```python
from build123d import *

# Parameters (mm, degrees)
SKETCH_3_W          = 4.4
SKETCH_3_H          = 18.2
EXTRUDE_1_DEPTH     = 1
SKETCH_4_R          = 0.95
CUT_EXTRUDE_1_DEPTH = 0.5
SKETCH_5_W          = 1
SKETCH_5_H          = 18.2
EXTRUDE_2_DEPTH     = 7
SKETCH_6_W          = 8.5
SKETCH_6_H          = 18.2
SKETCH_6_R          = 2
EXTRUDE_3_DEPTH     = 1
SKETCH_8_W          = 8.5
SKETCH_8_H          = 0.3
CUT_EXTRUDE_3_DEPTH = 0.2
SKETCH_9_R          = 0.6
CUT_EXTRUDE_4_DEPTH = 24.107989665
SKETCH_10_W         = 1
SKETCH_10_H         = 5.3
CUT_EXTRUDE_5_DEPTH = 2
FILLET_1_R          = 0.5


with BuildPart() as part:
    # 草圖3 → 填料-伸長1 (new body)
    with BuildSketch(Plane.XY):
        with Locations((3.460771452, 7.885973071)):
            Rectangle(SKETCH_3_W, SKETCH_3_H)
    extrude(amount=EXTRUDE_1_DEPTH)

    # 草圖4 → 除料-伸長1 (cut)
    with BuildSketch(Plane.XY.offset(1)):
        with Locations((3.460771452, 15.485973071)):
            Circle(SKETCH_4_R)
        with Locations((3.460771452, 0.285973071)):
            Circle(SKETCH_4_R)
        with Locations((3.460771452, 12.985973071)):
            Circle(SKETCH_4_R)
        with Locations((3.460771452, 2.785973071)):
            Circle(SKETCH_4_R)
    extrude(amount=-CUT_EXTRUDE_1_DEPTH, mode=Mode.SUBTRACT)

    # 草圖5 → 填料-伸長2 (add)
    with BuildSketch(Plane.XY.offset(1)):
        with Locations((5.160771452, 7.885973071)):
            Rectangle(SKETCH_5_W, SKETCH_5_H)
    extrude(amount=EXTRUDE_2_DEPTH)

    # 草圖6 → 填料-伸長3 (add)
    with BuildSketch(Plane.XY.offset(8)):
        with Locations((8.910771452, 7.885973071)):
            Rectangle(SKETCH_6_W, SKETCH_6_H)
        with Locations((9.254845598, 7.885973071)):
            Circle(SKETCH_6_R, mode=Mode.SUBTRACT)
    extrude(amount=EXTRUDE_3_DEPTH)

    # 草圖8 → 除料-伸長3 (cut)
    with BuildSketch(Plane.XY.offset(9)):
        with Locations((8.910771452, 7.885973071)):
            Rectangle(SKETCH_8_W, SKETCH_8_H)
    extrude(amount=-CUT_EXTRUDE_3_DEPTH, mode=Mode.SUBTRACT)

    # 草圖9 → 除料-伸長4 (cut, through all)
    with BuildSketch(Plane.XY.offset(0.5)):
        with Locations((3.460771452, 15.485973071)):
            Circle(SKETCH_9_R)
        with Locations((3.460771452, 12.985973071)):
            Circle(SKETCH_9_R)
        with Locations((3.460771452, 2.785973071)):
            Circle(SKETCH_9_R)
        with Locations((3.460771452, 0.285973071)):
            Circle(SKETCH_9_R)
    extrude(amount=-CUT_EXTRUDE_4_DEPTH, mode=Mode.SUBTRACT)

    # 草圖10 → 除料-伸長5 (cut)
    with BuildSketch(Plane.ZY.offset(-1.260771452)):
        with Locations((0.5, 7.885973071)):
            Rectangle(SKETCH_10_W, SKETCH_10_H)
    extrude(amount=-CUT_EXTRUDE_5_DEPTH, mode=Mode.SUBTRACT)

    # 圓角1
    fillet_1_edges = [part.edges().sort_by_distance(p)[0] for p in [
        (3.260771452, 5.235973071, 0.5),
        (3.260771452, 10.535973071, 0.5),
    ]]
    fillet(fillet_1_edges, radius=FILLET_1_R)


solid = part.part
```
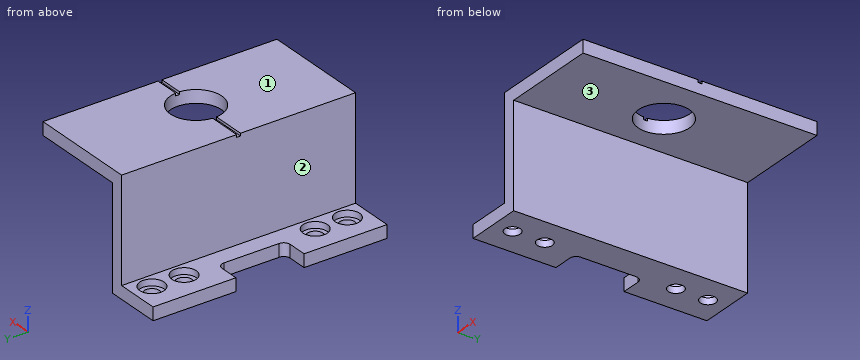
Part model, mm, in its own coordinate system. Face numbers are marked on the shaded views. A direction names the side the tool comes from. Round coordinates to 2 decimals unless told otherwise and drop trailing zeros. Write each loop counter-clockwise with the first axis right and the second up, starting at its lowest first coordinate (ties: lowest second). Pieces come first, ordered by that corner, then holes. Notation, with made-up numbers: M 53.25,42 L 72.25,42 A16 ccw 72.25,60 Z; hole C 70.25,2 d11. An arc over 180 degrees is marked long. Answer as CSV lines item,"result". Start each with the question number.
1) Drill centre lines: L1, parallel to X at y = 3.5, z = 7.25; L2, parallel to Z at x = 4.25, y = 4.75; L3, parallel to Z at x = 9.25, y = 5.5. Where is each one in solid material? Low to high.
2) Band-saw the part on C-C (z = 0.75). List the corners of the cut face in (x, y), then the cut area to 3 significant figures.
3) Band-saw the part on D-D (x = 6). List the corners of the cut face in (y, z), then the cut area to 3 significant figures.
4) Band-saw the part on B-B (y = 7.5). List the corners of the cut face in (x, z), then the cut area to 3 significant figures.
5) Drop flat-ended pins along their axis: pin 1 (2 mm diameter, centred on x = 9.5, y = 4.5, fed in from -Z); pin 2 (1.1 mm diameter, centred on x = 3.46, y = 0.29, fed in from -Z); pin 3 (4 mm diameter, centred on y = 3.5, z = 5.5, fed in from -X); pin 4 (2 mm diameter, centred on x = 3.5, y = 15, fed in from +Z). Give the stop position or say it passes through.
6) Band-saw the part on A-A (x = 9.25). List the corners of the cut face in (y, z).
7) Which spindle directions (+Z, -Z, +X, -X, +Y, -Y) get a long thin tool onto all of the face, cutting with end or side? Do the marked faces 1, 2 and 3. Say none if no direction does.
Worked out:
1,L1,"4.66 to 5.66"
1,L2,"0 to 1"
1,L3,"8 to 9"
2,outline,"M 1.26,-1.21 L 5.66,-1.21 L 5.66,16.99 L 1.26,16.99 L 1.26,10.54 L 2.76,10.54 A0.5 cw 3.26,10.04 L 3.26,5.74 A0.5 cw 2.76,5.24 L 1.26,5.24 Z; hole C 3.46,0.29 d1.9; hole C 3.46,2.79 d1.9; hole C 3.46,12.99 d1.9; hole C 3.46,15.49 d1.9"
2,area,"58.2 mm²"
3,outline,"M -1.21,8 L 16.99,8 L 16.99,9 L 8.04,9 L 8.04,8.8 L 7.74,8.8 L 7.74,9 L -1.21,9 Z"
3,area,"18.1 mm²"
4,outline,"M 3.26,0 L 5.66,0 L 5.66,8 L 7.29,8 L 7.29,9 L 4.66,9 L 4.66,1 L 3.26,1 Z; M 11.22,8 L 13.16,8 L 13.16,9 L 11.22,9 Z"
4,area,"14.0 mm²"
5,pin 1,"z = 8"
5,pin 2,"through"
5,pin 3,"x = 4.66"
5,pin 4,"z = 1"
6,outline,"M -1.21,8 L 5.89,8 L 5.89,9 L -1.21,9 Z; M 9.89,8 L 16.99,8 L 16.99,9 L 9.89,9 Z"
7,face 1,"+Z, +X, -X, +Y, -Y"
7,face 2,"+Z, -X, +Y, -Y"
7,face 3,"-Z, +X, +Y, -Y"
